Read the model definition and answer for the solid it produces. Units are mm, in the model's axes. Face numbers are marked on the shaded views. A direction names the side the tool comes from. Round coordinates to 2 decimals unless told otherwise and drop trailing zeros. Loops run counter-clockwise (first coordinate to the right, second up) from the corner with the lowest first, then second, coordinate; pieces in that order, holes last. Notation, with made-up numbers: (71.25, 62.25) - (106.25, 62.25) arc R25 ccw to (106.25, 76.25) - close; hole circle Ø4 at (-17, 33.5). An arc over 180 degrees is marked (long way). Answer as CSV lines item,"result".
```python
from build123d import *

# Parameters (mm, degrees)
F1_DEPTH = 5
F3_DEPTH = 2.5
F5_DEPTH = 25


with BuildPart() as f1:
    # F0 (on Top) → F1 (new body)
    with BuildSketch(Plane.XY):
        with BuildLine():
            ThreePointArc((-9.771052, 43.610957), (-1.575845, 0.293702), (-9.771052, -43.023552))
            Line((-9.771052, -43.023552), (4.098068, -43.7835))
            ThreePointArc((4.098068, -43.7835), (12.388804, -0.328701), (4.668032, 43.230977))
            Line((4.668032, 43.230977), (-9.771052, 43.610957))
        make_face()
    extrude(amount=F1_DEPTH)

    # F2 (on face) → F3 (join)
    with BuildSketch(Plane.XY.offset(5)):
        with BuildLine():
            ThreePointArc((-7.36353, 43.547601), (-6.846603, 42.282316), (-6.345194, 41.010802))
            Line((-6.345194, 41.010802), (3.505516, 41.010802))
            Line((3.505516, 41.010802), (2.697484, 43.258171))
            Line((2.697484, 43.258171), (0.835687, 43.33183))
            Line((0.835687, 43.33183), (-7.36353, 43.547601))
        make_face()
        with BuildLine():
            ThreePointArc((-6.597064, -40.326348), (-7.1427, -41.683608), (-7.70606, -43.033606))
            Line((-7.70606, -43.033606), (-0.661875, -43.522683))
            Line((-0.661875, -43.522683), (1.406391, -43.636012))
            Line((1.406391, -43.636012), (2.504335, -40.825053))
            Line((2.504335, -40.825053), (-6.597064, -40.326348))
        make_face()
    extrude(amount=F3_DEPTH)

    # F4 (on face) → F5 (cut)
    with BuildSketch(Plane.XY.offset(5)):
        with BuildLine():
            ThreePointArc((-4.045194, 41.010802), (2.951389, 0.25698), (-4.300509, -40.452186))
            Line((-4.300509, -40.452186), (0.192751, -40.698391))
            ThreePointArc((0.192751, -40.698391), (7.492519, 0.133214), (0.454806, 41.010802))
            Line((0.454806, 41.010802), (-4.045194, 41.010802))
        make_face()
    extrude(amount=-F5_DEPTH, mode=Mode.SUBTRACT)


solid = f1.part
```
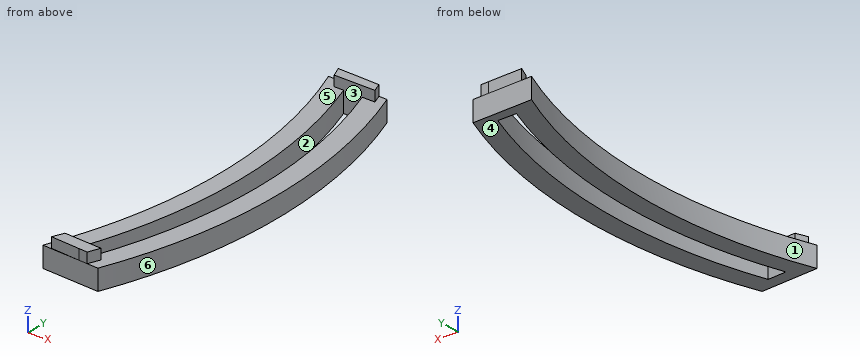
1) A cutting plane is placed at A-A, the plane z = 5.75. Determine the outline of the cut face in (x, y).
Entries:
outline,"(-7.71, -43.03) - (-0.66, -43.52) - (1.41, -43.64) - (2.5, -40.83) - (-6.6, -40.33) arc R111.72 cw to start; (-7.36, 43.55) arc R111.72 cw to (-6.35, 41.01) - (3.51, 41.01) - (2.7, 43.26) - (0.84, 43.33) - close"
2) A cutting plane is placed at D-D, the plane z = 1.5. Determine the outline of the cut face in (x, y), plus the area to 3 significant figures.
Entries:
outline,"(-9.77, -43.02) - (4.1, -43.78) arc R122.23 ccw to (4.67, 43.23) - (-9.77, 43.61) arc R118.58 cw to start; hole (-4.3, -40.45) - (0.19, -40.7) arc R120 ccw to (0.45, 41.01) - (-4.05, 41.01) arc R120 cw to start"
area,"849 mm^2"
3) A cutting plane is placed at C-C, the plane y = -10.5. Determine the outline of the cut face in (x, z), plus the area to 3 significant figures.
Entries:
outline,"(-2.07, 0) - (2.43, 0) - (2.43, 5) - (-2.07, 5) - close; (6.99, 0) - (11.9, 0) - (11.9, 5) - (6.99, 5) - close"
area,"47.1 mm^2"
4) Find the intervals of material crossed by line 1 (Y direction, x = -6, z = 6.75); line 2 (Z direction, x = 10, y = -18); line 3 (X direction, y = -23.5, z = 1), in increasing order.
Entries:
line 1,"y = -43.15 to -40.36, 41.01 to 43.51"
line 2,"z = 0 to 5"
line 3,"x = -3.99 to 0.5, 5.06 to 10.02"
5) A tool of negligible diameter and unlimited length cuts with its end or side. For the marked faces 1, 2 and 3, from which of +Z, -Z, +X, -X, +Y, -Y can it reach the whole face along a straight path? Write none if from no direction.
Entries:
face 1,"+Z, -Z, -X"
face 2,"+Z, -Z"
face 3,"+Z"
6) A cutting plane is placed at B-B, the plane y = -36. Determine the outline of the cut face in (x, z), plus the area to 3 significant figures.
Entries:
outline,"(-7.27, 0) - (-2.78, 0) - (-2.78, 5) - (-7.27, 5) - close; (1.8, 0) - (6.82, 0) - (6.82, 5) - (1.8, 5) - close"
area,"47.6 mm^2"
7) The mould has two halves that part along Y. Classify the marked faces 4, 5 and 6: pulls with the +Y half, pulls with the -Y half, needs draft (parallel to the pull), parting line crosses it, or undercut.
Entries:
face 4,"needs draft"
face 5,"undercut"
face 6,"parting line crosses it"
8) Each of these flat-tipped pins is pushed along its axis until it touches: P1, Ø12, axis at x = 3, y = 6, coming from the +Z side; P2, Ø4, axis at x = -2, z = 4, coming from the -Y side; P3, Ø4, axis at y = 6, z = 2.5, coming from the +X side. Where does it stop, or does it pass through?
Entries:
P1,"stops at z = 5"
P2,"stops at y = -43.56"
P3,"stops at x = 12.34"
